For this review, take the finished solid that the model builds, in its own axes (mm). Face numbers are marked on the shaded views. A direction names the side the tool comes from. Coordinates: 2 decimals unless noted, no trailing zeros. Loops run counter-clockwise (first coordinate to the right, second up) from the corner with the lowest first, then second, coordinate; pieces in that order, holes last. Notation, with made-up numbers: (11.5, 38.25) -> (27.5, 38.25) arc R32 ccw to (27.5, 67.25) -> close; hole circle Ø1 at (72.5, -36). An arc over 180 degrees is marked (long way). Answer in a Markdown table with one row per item.
from build123d import *

# Parameters (mm, degrees)
BOSS_EXTRUDE1_DEPTH = 14
SKETCH2_W           = 14
SKETCH2_H           = 12.5
BOSS_EXTRUDE2_DEPTH = 14
HOLE1_D             = 5


with BuildPart() as part:
    # Sketch1 → Boss-Extrude1 (new body)
    with BuildSketch(Plane(origin=(0, 0, 0), x_dir=(1, 0, 0), z_dir=(0, 1, 0))):
        with BuildLine():
            Line((-37.5, 12.5), (9.5, 12.5))
            ThreePointArc((9.5, 12.5), (12.5, 15.5), (15.5, 12.5))
            Line((15.5, 12.5), (25, 12.5))
            Line((25, 12.5), (25, 25))
            Line((25, 25), (0, 25))
            Line((0, 25), (-59.234271291, 112.5))
            Line((-59.234271291, 112.5), (-87.5, 112.5))
            Line((-87.5, 112.5), (-87.5, 87.5))
            Line((-87.5, 87.5), (-72.5, 87.5))
            Line((-72.5, 87.5), (-37.5, 35.798511432))
            Line((-37.5, 35.798511432), (-37.5, 12.5))
        make_face()
    extrude(amount=BOSS_EXTRUDE1_DEPTH)

    # Sketch2 → Boss-Extrude2 (add)
    with BuildSketch(Plane(origin=(0, 14, 0), x_dir=(1, 0, 0), z_dir=(0, 1, 0))):
        with Locations((-94.5, 100)):
            Rectangle(SKETCH2_W, SKETCH2_H)
    extrude(amount=-BOSS_EXTRUDE2_DEPTH)

    # Mirror1: part across plane


with BuildPart() as part_1:
    add(part.part)
    add(part.part.mirror(Plane(origin=(0, 14, -12.5), x_dir=(1, 0, 0), z_dir=(0, 0, -1))))

    # Hole1 (through all)
    with Locations(Plane(origin=(0, 14, 0), x_dir=(1, 0, 0), z_dir=(0, 1, 0))):
        with Locations((-64.234271291, 100), (-64.234271291, -75)):
            Hole(HOLE1_D / 2)


solid = part_1.part
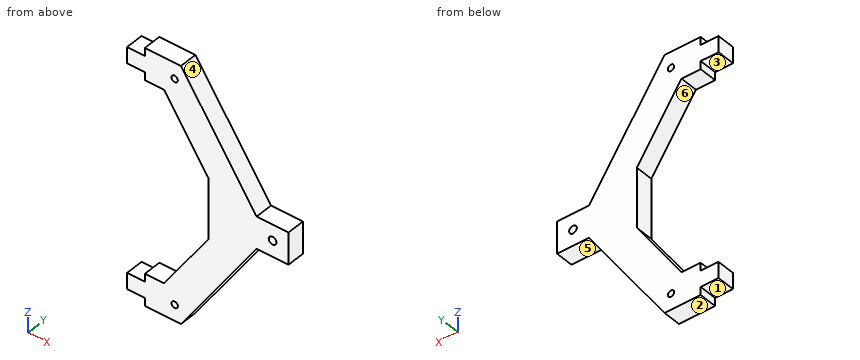
Item 1: For the marked faces 1, 2 and 3, list the 3-axis set-ups (+Z, -Z, +X, -X, +Y, -Y) from which the entire face can be reached by the end or side of a thin tool; tool diameter is ignored.
Worked answers:
| item | result |
|---|---|
| face 1 | -Z, -X, +Y, -Y |
| face 2 | -Z, +X, -X, +Y, -Y |
| face 3 | -X, +Y, -Y |
Item 2: The part is to be moulded in two halves that separate along Z. For the marked faces 4, 5 and 6, say which applies: +Z half, -Z half, draft (parallel to the pull), parting line (faces both ways), or undercut.
Worked answers:
| item | result |
|---|---|
| face 4 | +Z half |
| face 5 | -Z half |
| face 6 | undercut |
Item 3: Take a section at A-A, the plane x = 12.5. State the section outline as (y, z) points, and give its area (3 significant figures).
Worked answers:
| item | result |
|---|---|
| outline | (0, -25) -> (14, -25) -> (14, -15.5) -> (0, -15.5) -> close; (0, -9.5) -> (14, -9.5) -> (14, 0) -> (0, 0) -> close |
| area | 266 mm² |
Item 4: For L1, parallel to Z at x = -83.5, y = 9.25; L2, parallel to Z at x = 12.5, y = 4.5; L3, parallel to X at y = 12.25, z = -12, list the stretches that pass through material, from the lowest coordinate up.
Worked answers:
| item | result |
|---|---|
| L1 | -112.5 to -87.5, 62.5 to 87.5 |
| L2 | -25 to -15.5, -9.5 to 0 |
| L3 | -37.5 to 9.54, 15.46 to 25 |
Item 5: Insertion check: pin 1 (2 mm diameter, centred on y = 10.5, z = -52, fed in from -X); pin 2 (1.9 mm diameter, centred on y = 6, z = -89.5, fed in from -X); pin 3 (7 mm diameter, centred on x = 14, y = 6, fed in from +Z); pin 4 (4.5 mm diameter, centred on x = -64.23, z = 75, fed in from -Y). Each pin has a flat end and moves straight along its axis. Give the tip position at first contact, or say it passes through.
Worked answers:
| item | result |
|---|---|
| pin 1 | x = -49.14 |
| pin 2 | x = -87.5 |
| pin 3 | z = 0 |
| pin 4 | through |
Item 6: Take a section at B-B, the plane z = -12.5. State the section outline as (x, y) points.
Worked answers:
| item | result |
|---|---|
| outline | (-37.5, 0) -> (9.5, 0) -> (9.5, 14) -> (-37.5, 14) -> close; (15.5, 0) -> (25, 0) -> (25, 14) -> (15.5, 14) -> close |
Item 7: Take a section at C-C, the plane y = 9. State the section outline as (x, z) points, and give its area (3 significant figures).
Worked answers:
| item | result |
|---|---|
| outline | (-101.5, -106.25) -> (-87.5, -106.25) -> (-87.5, -112.5) -> (-59.23, -112.5) -> (0, -25) -> (25, -25) -> (25, 0) -> (0, 0) -> (-59.23, 87.5) -> (-87.5, 87.5) -> (-87.5, 81.25) -> (-101.5, 81.25) -> (-101.5, 68.75) -> (-87.5, 68.75) -> (-87.5, 62.5) -> (-72.5, 62.5) -> (-37.5, 10.8) -> (-37.5, -35.8) -> (-72.5, -87.5) -> (-87.5, -87.5) -> (-87.5, -93.75) -> (-101.5, -93.75) -> close; hole circle Ø5 at (-64.23, -100); hole circle Ø5 at (-64.23, 75); hole circle Ø6 at (12.5, -12.5) |
| area | 7,530 mm² |
Item 8: Take a section at D-D, the plane z = -81. State the section outline as (x, y) points, and give its area (3 significant figures).
Worked answers:
| item | result |
|---|---|
| outline | (-68.1, 0) -> (-37.91, 0) -> (-37.91, 14) -> (-68.1, 14) -> close |
| area | 423 mm² |
